from build123d import *

# Parameters (mm, degrees)
SKETCH1_W           = 38
SKETCH1_H           = 190
BOSS_EXTRUDE1_DEPTH = 1524
SKETCH2_W           = 190
SKETCH2_H           = 38
BOSS_EXTRUDE2_DEPTH = 190
CUT_EXTRUDE1_DEPTH  = 190


with BuildPart() as part:
    # Sketch1 → Boss-Extrude1 (new body)
    with BuildSketch(Plane(origin=(0, 0, 0), x_dir=(0, 0, -1), z_dir=(1, 0, 0))):
        Rectangle(SKETCH1_W, SKETCH1_H)
    extrude(amount=BOSS_EXTRUDE1_DEPTH)

    # Sketch2 → Boss-Extrude2 (add)
    with BuildSketch(Plane.XY.offset(19)):
        with Locations((95, -76)):
            Rectangle(SKETCH2_W, SKETCH2_H)
        with Locations((1429, -76)):
            Rectangle(SKETCH2_W, SKETCH2_H)
    extrude(amount=BOSS_EXTRUDE2_DEPTH)

    # Sketch3 → Cut-Extrude1 (cut)
    with BuildSketch(Plane(origin=(0, -57, 0), x_dir=(1, 0, 0), z_dir=(0, 1, 0))):
        Polygon((190, -19), (0, -209), (190, -209), align=None)
        Polygon((1334, -19), (1524, -209), (1334, -209), align=None)
    extrude(amount=-CUT_EXTRUDE1_DEPTH, mode=Mode.SUBTRACT)


solid = part.part
Source: CAD feature listing. Evaluate the final solid. Frame: model axes, mm. A direction names the side the tool comes from. Round coordinates to 2 decimals unless told otherwise and drop trailing zeros. Loops run counter-clockwise (first coordinate to the right, second up) from the corner with the lowest first, then second, coordinate; pieces in that order, holes last. Notation, with made-up numbers: (62, 34) -> (96, 34) arc R27 cw to (96, 70) -> close; hole circle Ø5 at (9.25, 82.25). An arc over 180 degrees is marked (long way). Answer as a JSON object with one key per item and string values. Group by question number.
Q1. Section query A-A (z = 82). Output: boundary loops of the cut face in (x, y).
Q2. Access query for faces 1 (the flat face through (1470, -57, 70)), 2 (the flat face through (751, -1, -19)), 3 (the flat face through (751, -1, 19)), 4 (the flat face through (96, -76, 113)). Directions: +Z, -Z, +X, -X, +Y, -Y. A direction counts if a zero-diameter tool reaches every point of the face in a straight line with its end or side. Return the directions, or none.
Q3. Section query B-B (z = 192). Output: boundary loops of the cut face in (x, y).
Q4. Ray query, line 1 (Z direction, x = 949, y = 39.5); line 2 (X direction, y = -59.5, z = 67); line 3 (X direction, y = -57.5, z = 68.5). Return the intervals inside material, ascending. Write a range as from..to.
Q5. Contact query for a flat-ended pin moving along its axis: P1, Ø10, axis at x = 202, y = 2.5, coming from the +Z side. Output: stop coordinate, or through.
Q6. Section query C-C (x = 1360.5). Output: boundary loops of the cut face in (y, z), plus the area to 3 significant figures.
Q7. Section query D-D (y = -30). Output: boundary loops of the cut face in (x, z).
Completed:
{
 "1": {"outline": "(0, -95) -> (127, -95) -> (127, -57) -> (0, -57) -> close; (1397, -95) -> (1524, -95) -> (1524, -57) -> (1397, -57) -> close"},
 "2": {"face 1": "+Z, +X, -X, +Y", "face 2": "-Z, +X, -X, +Y, -Y", "face 3": "+Z, +Y", "face 4": "+Z, +Y, -Y"},
 "3": {"outline": "(0, -95) -> (17, -95) -> (17, -57) -> (0, -57) -> close; (1507, -95) -> (1524, -95) -> (1524, -57) -> (1507, -57) -> close"},
 "4": {"line 1": "-19..19", "line 2": "0..142, 1382..1524", "line 3": "0..140.5, 1383.5..1524"},
 "5": {"P1": "z = 19"},
 "6": {"outline": "(-95, -19) -> (95, -19) -> (95, 19) -> (-57, 19) -> (-57, 45.5) -> (-95, 45.5) -> close", "area": "8,230 mm²"},
 "7": {"outline": "(0, -19) -> (1524, -19) -> (1524, 19) -> (0, 19) -> close"}
}
